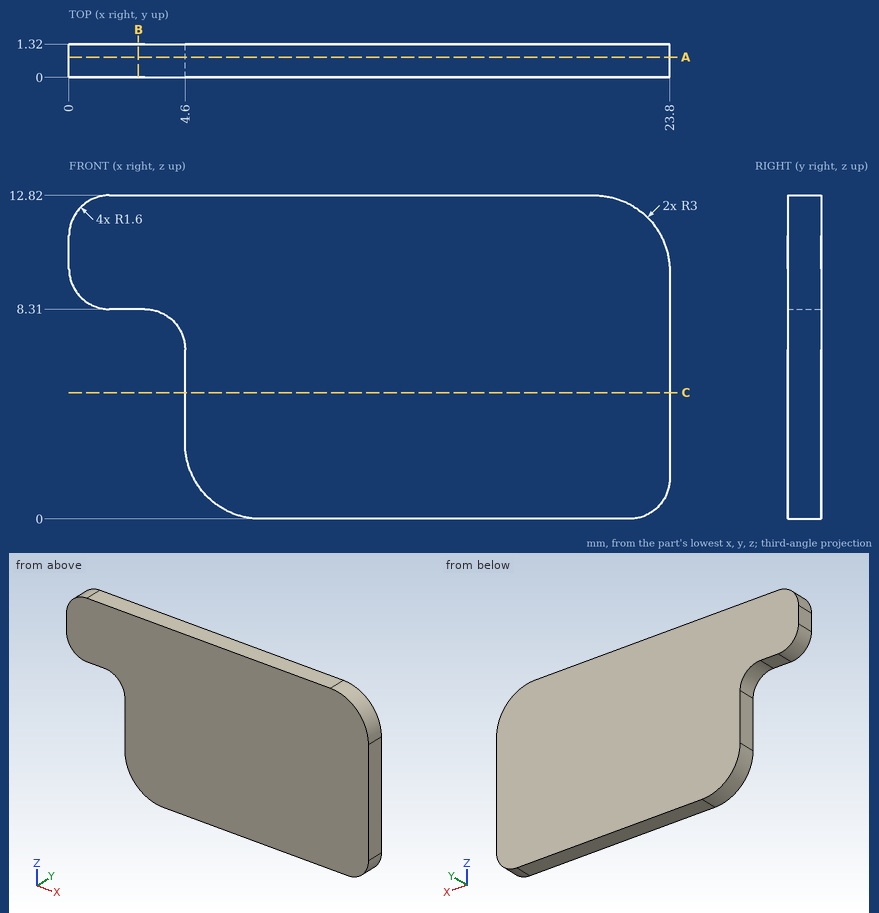
Could you check a few things on this drawing? It's one solid part, dimensions in mm from its lowest x, y, z. Round coordinates to 2 decimals unless told otherwise and drop trailing zeros. Order: outer loops, then holes, each group sorted by start corner. A loop starts at its lowest first (then second) coordinate and runs counter-clockwise, first axis right, second up.
Q1. Please list where these lines run through material, in increasing order: probe 1 along Z at (x, y) = (1.75, 0.2); probe 2 along X at (y, z) = (0.4, 5.25); probe 3 along X at (y, z) = (1.05, 12).
Geometry says:
probe 1: z = 8.31 to 12.82
probe 2: x = 4.6 to 23.8
probe 3: x = 0.2 to 22.86
Q2. Imagine slicing it at A-A, the plane y = 0.8. List the corners of the cut face in (x, z) for me.
Geometry says:
outline: (0, 9.91) arc R1.6 ccw to (1.6, 8.31) - (3, 8.31) arc R1.6 cw to (4.6, 6.71) - (4.6, 3) arc R3 ccw to (7.6, 0) - (22.2, 0) arc R1.6 ccw to (23.8, 1.6) - (23.8, 9.82) arc R3 ccw to (20.8, 12.82) - (1.6, 12.82) arc R1.6 ccw to (0, 11.22) - close
Q3. Imagine slicing it at B-B, the plane x = 2.75. List the corners of the cut face in (y, z) for me, then the cut area to 3 significant figures.
Geometry says:
outline: (0, 8.31) - (1.32, 8.31) - (1.32, 12.82) - (0, 12.82) - close
area: 5.95 mm2
Q4. Imagine slicing it at C-C, the plane z = 5. List the corners of the cut face in (x, y) for me.
Geometry says:
outline: (4.6, 0) - (23.8, 0) - (23.8, 1.32) - (4.6, 1.32) - close
